from build123d import *

# Parameters (mm, degrees)
F0_W     = 1
F0_H     = 0.5
F1_DEPTH = 16
F2_R     = 5


with BuildPart() as f1:
    # F0 (on Top) → F1 (new body)
    with BuildSketch(Plane.XY):
        Polygon((32.25, -2.5), (32.25, 2.5), (28.25, 2.5), (-28.25, 2.5), (-32.25, 2.5), (-32.25, -2.5), align=None)
        Polygon((32.25, 10.8), (32.25, 2.5), (32.25, -2.5), (32.25, -27.5), (39.25, -27.5), (39.25, 14.5), (32.25, 14.5), align=None)
        with BuildLine():
            ThreePointArc((28.55, 14.5), (30.1958719271, 12.4458719271), (32.25, 10.8))
            Line((32.25, 10.8), (32.25, 14.5))
            Line((32.25, 14.5), (28.55, 14.5))
        make_face()
        Polygon((27.25, 14.5), (28.25, 14.5), (28.55, 14.5), (32.25, 14.5), (39.25, 14.5), (39.25, 16), (26.25, 16), (26.25, 14.5), align=None)
        Polygon((-32.25, -27.5), (-32.25, -2.5), (-32.25, 2.5), (-39.25, 2.5), (-39.25, -27.5), align=None)
        Polygon((-39.25, 2.5), (-32.25, 2.5), (-32.25, 10.5), (-32.25, 10.8), (-32.25, 14.5), (-39.25, 14.5), align=None)
        with Locations((26.75, 14.25)):
            Rectangle(F0_W, F0_H)
        Polygon((-28.55, 14.5), (-28.25, 14.5), (-27.25, 14.5), (-26.25, 14.5), (-26.25, 16), (-39.25, 16), (-39.25, 14.5), (-32.25, 14.5), align=None)
        with BuildLine():
            Line((-32.25, 14.5), (-32.25, 10.8))
            ThreePointArc((-32.25, 10.8), (-31.7185283382, 11.1576250938), (-31.2068981187, 11.5431018813))
            Line((-31.2068981187, 11.5431018813), (-29.2931018813, 13.4568981187))
            ThreePointArc((-29.2931018813, 13.4568981187), (-28.9076250938, 13.9685283382), (-28.55, 14.5))
            Line((-28.55, 14.5), (-32.25, 14.5))
        make_face()
        with Locations((-26.75, 14.25)):
            Rectangle(F0_W, F0_H)
        with BuildLine():
            Line((-29.2931018813, 13.4568981187), (-31.2068981187, 11.5431018813))
            ThreePointArc((-31.2068981187, 11.5431018813), (-30.1958719271, 12.4458719271), (-29.2931018813, 13.4568981187))
        make_face()
    extrude(amount=F1_DEPTH)

    # F2
    f2_edges = [f1.edges().sort_by_distance(p)[0] for p in [
        (-39.25, 16, 8),
        (39.25, 16, 8),
    ]]
    fillet(f2_edges, radius=F2_R)


solid = f1.part
Source: CAD feature listing. Evaluate the final solid. Frame: model axes, mm. A direction names the side the tool comes from. Give positions to 0.01 mm unless a question says otherwise; leave off trailing zeros. Loops run counter-clockwise (first coordinate to the right, second up) from the corner with the lowest first, then second, coordinate; pieces in that order, holes last. Notation, with made-up numbers: (23.25, 66.5) -> (82.25, 66.5) arc R23 ccw to (82.25, 101.5) -> close; hole circle Ø3 at (39, -38). An arc over 180 degrees is marked (long way). Use a Markdown table: item, result. Add a question column.
1) Line query: line 1 along X through (y, z) = (-23, 8.25); line 2 along Y through (x, z) = (-32, 4.5); line 3 along Y through (x, z) = (-7, 8). Output: solid intervals per line, ascending. Write a range as [from, to].
2) Section query A-A, the plane y = -21. Return the cut outline in (x, z), then the cut area to 3 significant figures.
3) Pull-direction query (Y, two-part tool) for faces 1 (the face through (30.17, 12.47, 7.89)), 2 (the face through (-36, -27.5, 8)), 3 (the face through (39.25, -9, 8)); classes: +Y half, -Y half, draft (parallel to the pull), parting line (faces both ways), or undercut.
4) Section query B-B, the plane z = 14. Return the cut outline in (x, y), then the cut area to 3 significant figures.
5) Section query C-C, the plane x = -20. Return the cut outline in (y, z), then the cut area to 3 significant figures.
6) First-contact query: pin 1 (1.6 mm diameter, centred on y = 14.5, z = 7.5, fed in from +X); pin 2 (0.7 mm diameter, centred on x = 28, z = 5, fed in from -Y); pin 3 (1 mm diameter, centred on y = 15.5, z = 7.5, fed in from -X). Flat tips, straight axial feed; report the tip coordinate or a pass-through.
7) Reachability of faces 4 (the face through (-26.25, 15, 8)), 5 (the face through (32.25, 7, 8)), 6 (the face through (0, -2.5, 8)) from +Z, -Z, +X, -X, +Y, -Y: full face, straight path, thin tool, end or side. Return the list, or none.
Numbers:
| question | item | result |
|---|---|---|
| 1 | line 1 | x = [-39.25, -32.25], [32.25, 39.25] |
| 1 | line 2 | y = [-2.5, 2.5], [10.96, 16] |
| 1 | line 3 | y = [-2.5, 2.5] |
| 2 | outline | (-39.25, 0) -> (-32.25, 0) -> (-32.25, 16) -> (-39.25, 16) -> close; (32.25, 0) -> (39.25, 0) -> (39.25, 16) -> (32.25, 16) -> close |
| 2 | area | 224 mm2 |
| 3 | face 1 | undercut |
| 3 | face 2 | -Y half |
| 3 | face 3 | draft |
| 4 | outline | (-39.25, -27.5) -> (-32.25, -27.5) -> (-32.25, -2.5) -> (32.25, -2.5) -> (32.25, -27.5) -> (39.25, -27.5) -> (39.25, 11) arc R5 ccw to (34.25, 16) -> (26.25, 16) -> (26.25, 14) -> (27.25, 14) -> (27.25, 14.5) -> (28.55, 14.5) arc R12 ccw to (32.25, 10.8) -> (32.25, 2.5) -> (-32.25, 2.5) -> (-32.25, 10.8) arc R12 ccw to (-28.55, 14.5) -> (-27.25, 14.5) -> (-27.25, 14) -> (-26.25, 14) -> (-26.25, 16) -> (-34.25, 16) arc R5 ccw to (-39.25, 11) -> close |
| 4 | area | 955 mm2 |
| 5 | outline | (-2.5, 0) -> (2.5, 0) -> (2.5, 16) -> (-2.5, 16) -> close |
| 5 | area | 80.0 mm2 |
| 6 | pin 1 | stops at x = 38.46 |
| 6 | pin 2 | stops at y = -2.5 |
| 6 | pin 3 | stops at x = -37.25 |
| 7 | face 4 | +Z, -Z, +Y |
| 7 | face 5 | +Z, -Z |
| 7 | face 6 | +Z, -Z, -Y |
